Design review of the part built by this model. Coordinates are the model's own, in mm. Face numbers are marked on the shaded views. A direction names the side the tool comes from. Round coordinates to 2 decimals unless told otherwise and drop trailing zeros. Write each loop counter-clockwise with the first axis right and the second up, starting at its lowest first coordinate (ties: lowest second). Pieces come first, ordered by that corner, then holes. Notation, with made-up numbers: M 42,74 L 58,74 A24 cw 58,101 Z; hole C -36.5,23 d5. An arc over 180 degrees is marked long. Use CSV: the item, a comma, the result in double quotes.
from build123d import *

# Parameters (mm, degrees)
SALIENTE_EXTRUIR1_DEPTH = 18
SALIENTE_EXTRUIR2_START = 1.5
CROQUIS2_R              = 2.7
SALIENTE_EXTRUIR2_DEPTH = 1.5
SALIENTE_EXTRUIR3_DEPTH = 1.5
CROQUIS6_W              = 5.4
CROQUIS6_H              = 1.181933233
SALIENTE_EXTRUIR7_DEPTH = 10
CROQUIS7_W              = 5.4
CROQUIS7_H              = 10
CORTAR_EXTRUIR2_DEPTH   = 16.5
CROQUIS9_W              = 52.468080771
CROQUIS9_H              = 55.683263094
CORTAR_EXTRUIR3_DEPTH   = 30
CROQUIS10_W             = 2
CROQUIS10_H             = 3
CROQUIS10_W_2           = 2.00103554
CORTAR_EXTRUIR4_DEPTH   = 10
CROQUIS11_W             = 3.003829207
CROQUIS11_H             = 8.377286569
CROQUIS11_W_2           = 3
CROQUIS11_H_2           = 6.580683582
CORTAR_EXTRUIR5_DEPTH   = 7.4


with BuildPart() as part:
    # Croquis1 → Saliente-Extruir1 (new body)
    with BuildSketch(Plane.XY):
        with BuildLine():
            Line((-54.535099114, 31.482780649), (-55.25791247, 32.775048384))
            Line((-55.25791247, 32.775048384), (-58.679569293, 30.903614553))
            ThreePointArc((-58.679569293, 30.903614553), (-72.555259572, 38.768368337), (-85.712228427, 29.752642999))
            Line((-85.712228427, 29.752642999), (-86.469958437, 28.480534403))
            Line((-86.469958437, 28.480534403), (-83.138420786, 26.453009587))
            ThreePointArc((-83.138420786, 26.453009587), (-83.011652218, 10.503932418), (-68.625320614, 3.617525822))
            Line((-68.625320614, 3.617525822), (-67.144777249, 3.597366682))
            Line((-67.144777249, 3.597366682), (-67.054658077, 7.49632533))
            ThreePointArc((-67.054658077, 7.49632533), (-53.305736365, 15.580648714), (-54.535099114, 31.482780649))
        make_face()
        with BuildLine():
            Line((-69.624216052, 5.117649823), (-68.624216052, 5.117649823))
            Line((-68.624216052, 5.117649823), (-68.624216052, 9.117649823))
            ThreePointArc((-68.624216052, 9.117649823), (-55.305921191, 15.218525867), (-55.334796889, 29.867649823))
            Line((-55.334796889, 29.867649823), (-55.834796889, 30.733675227))
            Line((-55.834796889, 30.733675227), (-59.298898504, 28.733675227))
            ThreePointArc((-59.298898504, 28.733675227), (-71.241559574, 37.21721889), (-83.913635214, 29.867649823))
            Line((-83.913635214, 29.867649823), (-84.413635214, 29.001624419))
            Line((-84.413635214, 29.001624419), (-80.949533599, 27.001624419))
            ThreePointArc((-80.949533599, 27.001624419), (-82.325167391, 12.417204713), (-69.624216052, 5.117649823))
        make_face(mode=Mode.SUBTRACT)
    extrude(amount=SALIENTE_EXTRUIR1_DEPTH)

    # Croquis2 → Saliente-Extruir2 (add)
    with BuildSketch(Plane(origin=(0, 0, 0), x_dir=(-1, 0, 0), z_dir=(0, 0, -1)).offset(SALIENTE_EXTRUIR2_START)):
        with BuildLine():
            Line((67.054658077, 7.49632533), (67.144777249, 3.597366682))
            Line((67.144777249, 3.597366682), (68.625320614, 3.617525822))
            ThreePointArc((68.625320614, 3.617525822), (83.011652218, 10.503932418), (83.138420786, 26.453009587))
            Line((83.138420786, 26.453009587), (86.469958437, 28.480534403))
            Line((86.469958437, 28.480534403), (85.712228427, 29.752642999))
            ThreePointArc((85.712228427, 29.752642999), (72.555259572, 38.768368337), (58.679569293, 30.903614553))
            Line((58.679569293, 30.903614553), (55.25791247, 32.775048384))
            Line((55.25791247, 32.775048384), (54.535099114, 31.482780649))
            ThreePointArc((54.535099114, 31.482780649), (53.305736365, 15.580648714), (67.054658077, 7.49632533))
        make_face()
        with Locations((69.624216052, 21.617649823)):
            Circle(CROQUIS2_R, mode=Mode.SUBTRACT)
    extrude(amount=-SALIENTE_EXTRUIR2_DEPTH)

    # Croquis3 → Saliente-Extruir3 (add)
    with BuildSketch(Plane.XY.offset(18)):
        with BuildLine():
            Line((-67.144777249, 3.597366682), (-67.054658077, 7.49632533))
            ThreePointArc((-67.054658077, 7.49632533), (-53.305736365, 15.580648714), (-54.535099114, 31.482780649))
            Line((-54.535099114, 31.482780649), (-55.25791247, 32.775048384))
            Line((-55.25791247, 32.775048384), (-58.679569293, 30.903614553))
            ThreePointArc((-58.679569293, 30.903614553), (-72.555259572, 38.768368337), (-85.712228427, 29.752642999))
            Line((-85.712228427, 29.752642999), (-86.469958437, 28.480534403))
            Line((-86.469958437, 28.480534403), (-83.138420786, 26.453009587))
            ThreePointArc((-83.138420786, 26.453009587), (-83.011652218, 10.503932418), (-68.625320614, 3.617525822))
            Line((-68.625320614, 3.617525822), (-67.144777249, 3.597366682))
        make_face()
    extrude(amount=SALIENTE_EXTRUIR3_DEPTH)

    # Croquis6 → Saliente-Extruir7 (add)
    with BuildSketch(Plane(origin=(0, 0, -1.5), x_dir=(-1, 0, 0), z_dir=(0, 0, -1))):
        with Locations((69.624216052, 21.026683207)):
            Rectangle(CROQUIS6_W, CROQUIS6_H)
    extrude(amount=SALIENTE_EXTRUIR7_DEPTH)

    # Croquis7 → Cortar-Extruir2 (cut)
    with BuildSketch(Plane(origin=(0, 21.617649823, 0), x_dir=(1, 0, 0), z_dir=(0, 1, 0))):
        with Locations((-69.624216052, 6.5)):
            Rectangle(CROQUIS7_W, CROQUIS7_H)
    extrude(amount=-CORTAR_EXTRUIR2_DEPTH, mode=Mode.SUBTRACT)

    # Croquis8 → Revolución1 (revolve)
    with BuildSketch(Plane(origin=(0, 21.617649823, 0), x_dir=(1, 0, 0), z_dir=(0, 1, 0)), mode=Mode.PRIVATE) as revoluci_n1_sk:
        Polygon((-72.324216052, 1.5), (-79.486781688, 1.5), (-72.324216052, 11.5), align=None)
        Polygon((-72.324216052, -19.5), (-69.624216052, -19.5), (-69.624216052, -25.5), (-72.324216052, -25.5), (-77.324216052, -25.5), (-77.324216052, -19.5), align=None)
    revolve(revoluci_n1_sk.sketch.rotate(Axis((-69.624216052, 21.617649823, 19.5), (0, 0, 1)), 180), axis=Axis((-69.624216052, 21.617649823, 19.5), (0, 0, 1)))

    # Croquis9 → Cortar-Extruir3 (cut)
    with BuildSketch(Plane(origin=(0, 21.617649823, 0), x_dir=(1, 0, 0), z_dir=(0, 1, 0))):
        with Locations((-61.70964897, -8.735329994)):
            Rectangle(CROQUIS9_W, CROQUIS9_H)
    extrude(amount=CORTAR_EXTRUIR3_DEPTH, mode=Mode.SUBTRACT)

    # Croquis10 → Cortar-Extruir4 (cut)
    with BuildSketch(Plane(origin=(0, 21.617649823, 0), x_dir=(1, 0, 0), z_dir=(0, 1, 0))):
        with Locations((-74.324216052, 4)):
            Rectangle(CROQUIS10_W, CROQUIS10_H)
        with Locations((-64.923698282, 4)):
            Rectangle(CROQUIS10_W_2, CROQUIS10_H)
        with Locations((-74.324216052, -22.35)):
            Rectangle(CROQUIS10_W, CROQUIS10_H)
        with Locations((-64.923698282, -22.35)):
            Rectangle(CROQUIS10_W_2, CROQUIS10_H)
    extrude(amount=-CORTAR_EXTRUIR4_DEPTH, mode=Mode.SUBTRACT)

    # Croquis11 → Cortar-Extruir5 (cut)
    with BuildSketch(Plane(origin=(-65.924216052, 0, 0), x_dir=(0, 0, -1), z_dir=(1, 0, 0))):
        with Locations((-22.348085397, 13.363371819)):
            Rectangle(CROQUIS11_W, CROQUIS11_H)
        with Locations((4, 12.973671933)):
            Rectangle(CROQUIS11_W_2, CROQUIS11_H_2)
    extrude(amount=-CORTAR_EXTRUIR5_DEPTH, mode=Mode.SUBTRACT)


solid = part.part
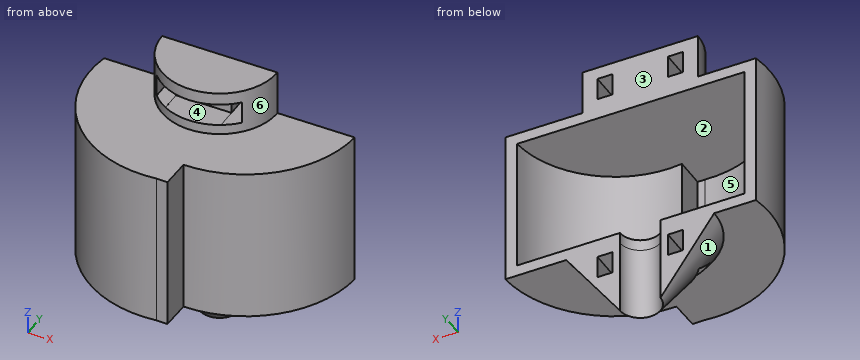
1) Add section D-D on y = 10.25. Write out the cut boundary in (x, z) (3 decimals).
Answers:
outline,"M -82.847,-1.5 L -57.966,-1.5 L -57.966,19.5 L -82.847,19.5 Z; hole M -80.927,0 L -60.985,0 L -60.985,18 L -80.927,18 Z"
2) For pin 1 Ø9 at (x, y) = (-61, 9) entering from +Z; pin 2 Ø3 at (y, z) = (7, 10.5) entering from -X; pin 3 Ø3.5 at (y, z) = (19, -4) entering from -X, all flat-tipped, find the tip position at first contact; note any pin that passes through.
Answers:
pin 1,"z = 19.5"
pin 2,"x = -81.49"
pin 3,"x = -78.65"
3) Add section A-A on z = -1. Write out the cut boundary in (x, y), then the cut area to 3 significant figures.
Answers:
outline,"M -85.05,21.62 A15.06 ccw -68.63,3.62 L -67.14,3.6 L -67.05,7.5 A15.06 ccw -51.63,21.62 L -66.92,21.62 A2.7 cw -72.32,21.62 Z"
area,"440 mm²"
4) Add section B-B on y = 6. Write out the cut boundary in (x, z), then the cut area to 3 significant figures.
Answers:
outline,"M -78.58,-1.5 L -67.09,-1.5 L -67.09,19.5 L -78.58,19.5 Z; hole M -75.15,0 L -68.62,0 L -68.62,18 L -75.15,18 Z"
area,"124 mm²"
5) Add section C-C on x = -57.5. Write out the cut boundary in (y, z).
Answers:
outline,"M 10.59,-1.5 L 21.62,-1.5 L 21.62,0 L 12.59,0 L 12.59,18 L 21.62,18 L 21.62,19.5 L 10.59,19.5 Z"
6) Wall thickness on line 1 along Z through (x, y) = (-75, 16.75); line 2 along Z through (x, y) = (-59, 17); line 3 along Z through (x, y) = (-65, 15): over which ranges is each line inside the solid? List them lowest first. Write a range as [from, to].
Answers:
line 1,"[-2.5, 0], [18, 20.85], [23.85, 25.5]"
line 2,"[-1.5, 0], [18, 19.5]"
line 3,"[-2.5, 0], [18, 19.5]"
7) Machinability: for the marked faces 4, 5 and 6, which of the approach directions +Z, -Z, +X, -X, +Y, -Y give a long, thin tool a straight path to every point of the face, cutting with its end or side? Answer none if there is none.
Answers:
face 4,"-Y"
face 5,"none"
face 6,"+Z, -Y"
8) The part is to be moulded in two halves that separate along X. For the marked faces 1, 2 and 3, say which applies: released by +X, released by -X, zero draft, split by the parting line, or undercut.
Answers:
face 1,"split by the parting line"
face 2,"undercut"
face 3,"zero draft"
